Geometry: final body of the model. Coordinates: model frame, mm. Face numbers are marked on the shaded views. A direction names the side the tool comes from. Give positions to 0.01 mm unless a question says otherwise; leave off trailing zeros. Write each loop counter-clockwise with the first axis right and the second up, starting at its lowest first coordinate (ties: lowest second). Pieces come first, ordered by that corner, then holes. Notation, with made-up numbers: (9.25, -10.75) -> (34.25, -10.75) arc R21 ccw to (34.25, 10.25) -> close; hole circle Ø7 at (4.25, 48). An arc over 180 degrees is marked (long way). Answer in a Markdown table with one row per item. Add a question column.
Item 1: Section query C-C on y = 8.5. Output: boundary loops of the cut face in (x, z), plus the area to 3 significant figures.
Item 2: Draft query along Z for the marked faces 1, 2 and 3. Return one class per face: +Z half, -Z half, draft (parallel to the pull), parting line (faces both ways), or undercut.
Item 3: Material intervals for probe 1 along Z at (x, y) = (4, -9.75); probe 2 along Z at (x, y) = (4, -3.25); probe 3 along Z at (x, y) = (6.75, -10), sorted ascending. Write a range as from..to.
Item 4: Section query B-B on z = -1. Output: boundary loops of the cut face in (x, y), plus the area to 3 significant figures.
Item 5: First-contact query: P1, Ø2, axis at x = 1.5, z = -1, coming from the +Y side; P2, Ø3, axis at x = 8, y = -5.5, coming from the -Z side; P3, Ø3, axis at x = 6.5, y = 19, coming from the +Z side; P4, Ø2, axis at x = 4, z = 22.11, coming from the +Y side. Flat tips, straight axial feed; report the tip coordinate or a pass-through.
Item 6: Section query A-A on y = -12. Output: boundary loops of the cut face in (x, z), plus the area to 3 significant figures.
Item 7: Section query D-D on x = 4. State how many separate pieces and enclosed holes the cut face has, plus the area to 3 significant figures.
Item 8: Access query for the marked faces 4 and 5. Directions: +Z, -Z, +X, -X, +Y, -Y. A direction counts if a zero-diameter tool reaches every point of the face in a straight line with its end or side. Return the directions, or none.
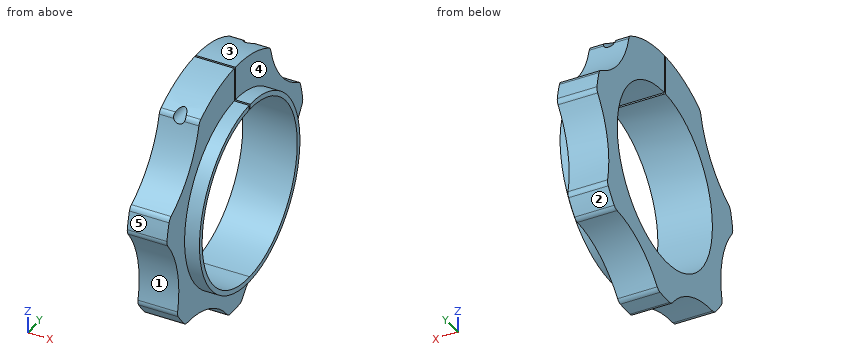
```python
from build123d import *

# Parameters (mm, degrees)
CROQUIS1_R              = 18
SALIENTE_EXTRUIR1_DEPTH = 8
CROQUIS2_R              = 19
CROQUIS2_R_2            = 18
SALIENTE_EXTRUIR2_DEPTH = 3
CROQUIS3_W              = 33
CROQUIS3_H              = 0.4
CORTAR_EXTRUIR2_DEPTH   = 16.5
REDONDEO1_R             = 1.5
CROQUIS4_R              = 1.190625
CORTAR_EXTRUIR3_DEPTH   = 16.5


with BuildPart() as part:
    # Croquis1 → Saliente-Extruir1 (new body)
    with BuildSketch(Plane(origin=(0, 0, 0), x_dir=(0, 0, -1), z_dir=(1, 0, 0))):
        with BuildLine():
            ThreePointArc((-22.245034297, 13.459511474), (-26, 0), (-22.245034297, -13.459511474))
            ThreePointArc((-22.245034297, -13.459511474), (-13.874638854, -17.398246822), (-8.172067613, -24.682327908))
            ThreePointArc((-8.172067613, -24.682327908), (-5.785544283, -25.348125717), (-3.346482217, -25.783736284))
            ThreePointArc((-3.346482217, -25.783736284), (4.951801275, -21.695258927), (14.202220202, -21.778359473))
            ThreePointArc((14.202220202, -21.778359473), (16.210734848, -20.327618544), (18.072039228, -18.69228178))
            ThreePointArc((18.072039228, -18.69228178), (20.049434046, -9.655298558), (25.881946532, -2.474842158))
            ThreePointArc((25.881946532, -2.474842158), (26, 0), (25.881946532, 2.474842158))
            ThreePointArc((25.881946532, 2.474842158), (20.049434046, 9.655298558), (18.072039228, 18.69228178))
            ThreePointArc((18.072039228, 18.69228178), (16.210734848, 20.327618544), (14.202220202, 21.778359473))
            ThreePointArc((14.202220202, 21.778359473), (4.951801275, 21.695258927), (-3.346482217, 25.783736284))
            ThreePointArc((-3.346482217, 25.783736284), (-5.785544283, 25.348125717), (-8.172067613, 24.682327908))
            ThreePointArc((-8.172067613, 24.682327908), (-13.874638854, 17.398246822), (-22.245034297, 13.459511474))
        make_face()
        Circle(CROQUIS1_R, mode=Mode.SUBTRACT)
    extrude(amount=SALIENTE_EXTRUIR1_DEPTH)

    # Croquis2 → Saliente-Extruir2 (add)
    with BuildSketch(Plane(origin=(8, 0, 0), x_dir=(0, 0, -1), z_dir=(1, 0, 0))):
        Circle(CROQUIS2_R)
        Circle(CROQUIS2_R_2, mode=Mode.SUBTRACT)
    extrude(amount=SALIENTE_EXTRUIR2_DEPTH)

    # Croquis3 → Cortar-Extruir2 (cut, symmetric)
    with BuildSketch(Plane(origin=(0, 0, 0), x_dir=(0, 0, -1), z_dir=(1, 0, 0))):
        with Locations((-16.5, 0)):
            Rectangle(CROQUIS3_W, CROQUIS3_H)
    extrude(amount=CORTAR_EXTRUIR2_DEPTH, both=True, mode=Mode.SUBTRACT)

    # Redondeo1
    redondeo1_edges = [part.edges().sort_by_distance(p)[0] for p in [
        (4, 25.783736284, 3.346482217),
        (4, 21.778359473, -14.202220202),
        (4, 18.69228178, -18.072039228),
        (4, 2.474842158, -25.881946532),
        (4, -2.474842158, -25.881946532),
        (4, -18.69228178, -18.072039228),
        (4, -21.778359473, -14.202220202),
        (4, -25.783736284, 3.346482217),
        (4, -24.682327908, 8.172067613),
        (4, -13.459511474, 22.245034297),
        (4, 13.459511474, 22.245034297),
        (4, 24.682327908, 8.172067613),
    ]]
    fillet(redondeo1_edges, radius=REDONDEO1_R)

    # Croquis4 → Cortar-Extruir3 (cut, symmetric)
    with BuildSketch(Plane.XZ.offset(-0.2)):
        with Locations(Location((4, 22.109052571, 0), (0, 0, 270))):
            Circle(CROQUIS4_R)
    extrude(amount=CORTAR_EXTRUIR3_DEPTH, both=True, mode=Mode.SUBTRACT)


solid = part.part
```
Findings below:
| question | item | result |
|---|---|---|
| 1 | outline | (0, -20.65) -> (8, -20.65) -> (8, -16.99) -> (11, -16.99) -> (11, -15.87) -> (0, -15.87) -> close; (0, 15.87) -> (11, 15.87) -> (11, 16.99) -> (8, 16.99) -> (8, 24.57) -> (0, 24.57) -> close; hole circle Ø2.38 at (4, 22.11) |
| 1 | area | 110 mm^2 |
| 2 | face 1 | undercut |
| 2 | face 2 | -Z half |
| 2 | face 3 | +Z half |
| 3 | probe 1 | z = -20..-15.13, 15.13..20.92, 23.3..24.1 |
| 3 | probe 2 | z = -24.93..-17.7, 17.7..20.92, 23.3..25.8 |
| 3 | probe 3 | z = -19.89..-14.97, 14.97..24 |
| 4 | outline | (0, -23.04) -> (8, -23.04) -> (8, -18.97) -> (11, -18.97) -> (11, -17.97) -> (0, -17.97) -> close; (0, 17.97) -> (11, 17.97) -> (11, 18.97) -> (8, 18.97) -> (8, 23.04) -> (0, 23.04) -> close |
| 4 | area | 87.2 mm^2 |
| 5 | P1 | stops at y = 23.54 |
| 5 | P2 | stops at z = -24.12 |
| 5 | P3 | stops at z = 13.75 |
| 5 | P4 | passes through |
| 6 | outline | (0, -19.1) -> (8, -19.1) -> (8, -14.73) -> (11, -14.73) -> (11, -13.42) -> (0, -13.42) -> close; (0, 13.42) -> (11, 13.42) -> (11, 14.73) -> (8, 14.73) -> (8, 23.07) -> (4.71, 23.07) arc R1.19 cw (long way) to (3.29, 23.07) -> (0, 23.07) -> close |
| 6 | area | 126 mm^2 |
| 7 | separate pieces | 3 |
| 7 | enclosed holes | 0 |
| 7 | area | 768 mm^2 |
| 8 | face 4 | +X |
| 8 | face 5 | +Z, +X, -X, -Y |
